Check sheet for the modelled part. Datum: model origin and axes. Units: mm. A direction names the side the tool comes from. Round coordinates to 2 decimals unless told otherwise and drop trailing zeros. Write each loop counter-clockwise with the first axis right and the second up, starting at its lowest first coordinate (ties: lowest second). Pieces come first, ordered by that corner, then holes.
from build123d import *

# Parameters (mm, degrees)
ESQUISSE1_W             = 80.3
ESQUISSE1_H             = 12.7
BOSS_EXTRU_1_DEPTH      = 12.7
ESQUISSE2_R             = 2.1
ESQUISSE2_R_2           = 1.6
ENL_V_MAT_EXTRU_1_DEPTH = 12.7
ENL_V_MAT_EXTRU_2_DEPTH = 12.7


with BuildPart() as part:
    # Esquisse1 → Boss.-Extru.1 (new body)
    with BuildSketch(Plane(origin=(0, 0, 0), x_dir=(1, 0, 0), z_dir=(0, 1, 0))):
        with Locations((40.15, -6.35)):
            Rectangle(ESQUISSE1_W, ESQUISSE1_H)
    extrude(amount=BOSS_EXTRU_1_DEPTH)

    # Esquisse2 → Enlèv. mat.-Extru.1 (cut)
    with BuildSketch(Plane(origin=(0, 12.7, 0), x_dir=(1, 0, 0), z_dir=(0, 1, 0))):
        with Locations((5.1, -6.35)):
            Circle(ESQUISSE2_R)
        with Locations((19.9, -6.35)):
            Circle(ESQUISSE2_R)
        with Locations((59.7, -6.35)):
            Circle(ESQUISSE2_R_2)
        with Locations((75.1, -6.35)):
            Circle(ESQUISSE2_R_2)
    extrude(amount=-ENL_V_MAT_EXTRU_1_DEPTH, mode=Mode.SUBTRACT)

    # Esquisse3 → Enlèv. mat.-Extru.2 (cut)
    with BuildSketch(Plane.XY.offset(12.7)):
        with BuildLine():
            ThreePointArc((38.67125, 7.057070345), (27.55, 6.121229313), (38.67125, 5.185388281))
            ThreePointArc((38.67125, 5.185388281), (40.15, 4.371229313), (41.62875, 5.185388281))
            ThreePointArc((41.62875, 5.185388281), (52.75, 6.121229313), (41.62875, 7.057070345))
            ThreePointArc((41.62875, 7.057070345), (40.15, 7.871229313), (38.67125, 7.057070345))
        make_face()
    extrude(amount=-ENL_V_MAT_EXTRU_2_DEPTH, mode=Mode.SUBTRACT)


solid = part.part
1. Release check for a two-part mould opening along Z. For faces 1 (the cylindrical face through (58.1, 6.4, 6.3)), 2 (the flat face through (40, 9, 0)), 3 (the flat face through (80.3, 6, 6)) record: released by +Z, released by -Z, zero draft, split by the parting line, or undercut.
2. Sectioned sample at A-A, the plane z = 6.35. Enter the section's corners in (x, y).
3. Go/stop test with a flat-tipped pin: pin 1 (1.5 mm diameter, centred on x = 34.5, y = 3.5, fed in from -Z). Record where the tip stops, or that it passes through.
4. Sectioned sample at B-B, the plane x = 47.15. Enter the section's corners in (y, z), plus the area to 4 significant figures.
5. Sectioned sample at C-C, the plane z = 2.75. Enter the section's corners in (x, y), plus the area to 3 significant figures.
6. Scan lines: line 1 along Y through (x, z) = (33.15, 10); line 2 along Z through (x, y) = (75.1, 9); line 3 along X through (y, z) = (9.25, 11.75). Record each from-to range of solid material in increasing order.
7. Set-up check for faces 4 (the cylindrical face through (40.13, 4.37, 6.44)), 5 (the cylindrical face through (4.64, 6.44, 8.4)): record each of +Z, -Z, +X, -X, +Y, -Y from which the full face is reachable in a straight line by a thin tool's end or side.
8. Sectioned sample at D-D, the plane x = 19.9. Enter the section's corners in (y, z), plus the area to 3 significant figures.
Computed values:
1. face 1: undercut
1. face 2: released by -Z
1. face 3: zero draft
2. outline: (0, 0) - (3, 0) - (3, 12.7) - (0, 12.7) - close; (7.2, 0) - (17.8, 0) - (17.8, 12.7) - (7.2, 12.7) - close; (22, 0) - (58.1, 0) - (58.1, 12.7) - (22, 12.7) - close; (61.3, 0) - (73.5, 0) - (73.5, 12.7) - (61.3, 12.7) - close; (76.7, 0) - (80.3, 0) - (80.3, 12.7) - (76.7, 12.7) - close; hole (38.67, 5.19) arc R1.75 ccw to (41.63, 5.19) arc R5.6 ccw (long way) to (41.63, 7.06) arc R1.75 ccw to (38.67, 7.06) arc R5.6 ccw (long way) to start
3. pin 1: passes through
4. outline: (0, 0) - (0.52, 0) - (0.52, 12.7) - (0, 12.7) - close; (11.72, 0) - (12.7, 0) - (12.7, 12.7) - (11.72, 12.7) - close
4. area: 19.05 mm2
5. outline: (0, 0) - (80.3, 0) - (80.3, 12.7) - (0, 12.7) - close; hole (38.67, 5.19) arc R1.75 ccw to (41.63, 5.19) arc R5.6 ccw (long way) to (41.63, 7.06) arc R1.75 ccw to (38.67, 7.06) arc R5.6 ccw (long way) to start
5. area: 814 mm2
6. line 1: y = 0 to 0.52, 11.72 to 12.7
6. line 2: z = 0 to 4.75, 7.95 to 12.7
6. line 3: x = 0 to 28.51, 37.79 to 42.51, 51.79 to 80.3
7. face 4: +Z, -Z
7. face 5: +Y, -Y
8. outline: (0, 0) - (12.7, 0) - (12.7, 4.25) - (0, 4.25) - close; (0, 8.45) - (12.7, 8.45) - (12.7, 12.7) - (0, 12.7) - close
8. area: 108 mm2
